Build history of the part. All positions in model axes, mm. Face numbers are marked on the shaded views. A direction names the side the tool comes from. Round coordinates to 2 decimals unless told otherwise and drop trailing zeros. Order: outer loops, then holes, each group sorted by start corner. A loop starts at its lowest first (then second) coordinate and runs counter-clockwise, first axis right, second up. Notation, with made-up numbers: M -27.75,31.5 L -1.75,31.5 A28 ccw -1.75,55.5 Z; hole C 35.25,84.25 d2. An arc over 180 degrees is marked long. One line per item, written item: value. Start each with the question number.
Item 1: Tool access for the marked faces 1, 2 and 3: list every direction of +Z, -Z, +X, -X, +Y, -Y with a clear straight run to the whole face (end or side of a thin tool).
Item 2: Pin check, flat tips, straight feed: pin 1 (5 mm diameter, centred on y = 14.5, z = 9.5, fed in from -X); pin 2 (2 mm diameter, centred on x = 9.5, z = 15.5, fed in from +Y); pin 3 (10 mm diameter, centred on y = 1, z = 11, fed in from +X). Stop position of each tip, or through.
Item 3: Probe L1, parallel to X at y = 17.5, z = 2; L2, parallel to X at y = 1.5, z = 9.75; L3, parallel to Z at x = 0.9, y = 25. List the from-to ranges inside material, lowest first.
Item 4: Two-plate mould, pull along Y, no slides. Class the marked faces 4, 5, 6 and 7: +Y half, -Y half, draft (parallel to the pull), parting line (faces both ways), or undercut.
Item 5: Band-saw the part on A-A, the plane x = 0. Write the cut outline in (y, z) (3 decimals).
Item 6: Band-saw the part on B-B, the plane y = 0. Write the cut outline in (x, z) (3 decimals), then the cut area to 3 significant figures.
Item 7: Band-saw the part on C-C, the plane y = 25. Write the cut outline in (x, z), then the cut area to 3 significant figures.
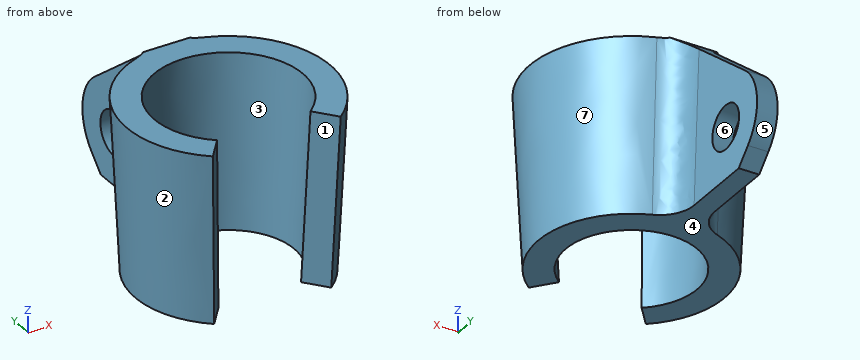
```python
from build123d import *

# Parameters (mm, degrees)
F1_ANGLE_BACK = 141
F1_ANGLE      = 282
F2_R          = 3.2
F3_DEPTH      = 1.5
F4_R          = 5


with BuildPart() as f1:
    # F0 (on Right) → F1 (revolve)
    with BuildSketch(Plane.YZ, mode=Mode.PRIVATE) as f1_sk:
        Polygon((9.6, 0), (13.6049968789, 0), (14.8549968789, 25), (10.85, 25), align=None)
    revolve(f1_sk.sketch.rotate(Axis((0, 0, 12.5), (0, 0, 1)), -F1_ANGLE_BACK), axis=Axis((0, 0, 12.5), (0, 0, 1)), revolution_arc=F1_ANGLE)

    # F2 (on Right) → F3 (join, symmetric)
    with BuildSketch(Plane.YZ):
        with BuildLine():
            Line((14.8549968789, 25), (10.85, 25))
            Line((10.85, 25), (9.6, 0))
            Line((9.6, 0), (25, 0))
            Line((25, 0), (28.1066017178, 0))
            Line((28.1066017178, 0), (30.3033008589, 2.1966991411))
            ThreePointArc((30.3033008589, 2.1966991411), (32.4865458897, 7.9490330074), (29.6313916174, 13.3991704236))
            Line((29.6313916174, 13.3991704236), (14.8549968789, 25))
        make_face()
        with Locations((25, 7.5)):
            Circle(F2_R, mode=Mode.SUBTRACT)
    extrude(amount=F3_DEPTH, both=True)

    # F4 (call 1 of 2: OpenCascade refuses the feature's edges together)
    f4_edges = [f1.edges().sort_by_distance(p)[0] for p in [
        (1.5, 14.150717, 12.499992),
    ]]
    fillet(f4_edges, radius=F4_R)

    # F4#2 (call 2 of 2)
    f4_2_edges = [f1.edges().sort_by_distance(p)[0] for p in [
        (-1.5, 14.150717, 12.499992),
    ]]
    fillet(f4_2_edges, radius=F4_R)


solid = f1.part
```
Output:
1. face 1: +Z, -Z, -Y
1. face 2: -Z, -X
1. face 3: +Z
2. pin 1: stops at x = -7.37
2. pin 2: stops at y = 11.6
2. pin 3: stops at x = 14.4
3. L1: x = -1.5 to 1.5
3. L2: x = -14.01 to -9.98, 9.98 to 14.01
3. L3: z = 0 to 4.3, 10.7 to 17.04
4. face 4: draft
4. face 5: +Y half
4. face 6: undercut
4. face 7: parting line
5. outline: M 9.6,0 L 28.107,0 L 30.303,2.197 A7.5 ccw 29.631,13.399 L 14.855,25 L 10.85,25 Z; hole C 25,7.5 d6.4
6. outline: M -14.855,25 L -13.605,0 L -9.6,0 L -10.85,25 Z; M 9.6,0 L 13.605,0 L 14.855,25 L 10.85,25 Z
6. area: 200 mm²
7. outline: M -1.5,0 L 1.5,0 L 1.5,4.3 L -1.5,4.3 Z; M -1.5,10.7 L 1.5,10.7 L 1.5,17.04 L -1.5,17.04 Z
7. area: 31.9 mm²
